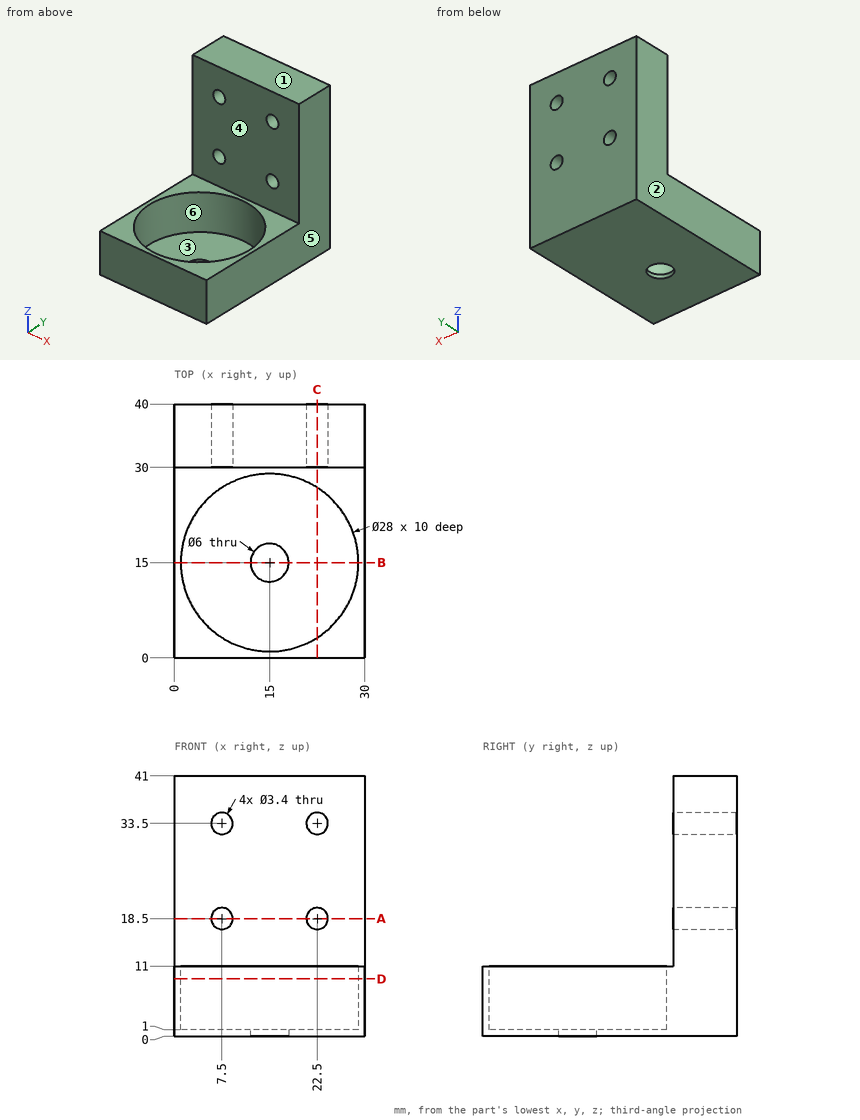
Drawing for the job (mm, zero at the part's lowest x, y, z). A direction names the side the tool comes from. Give positions to 0.01 mm unless a question says otherwise; leave off trailing zeros. Loops run counter-clockwise (first coordinate to the right, second up) from the corner with the lowest first, then second, coordinate; pieces in that order, holes last.
Item 1: Mould opens along X. For the marked faces 1, 2 and 3 say: +X half, -X half, draft (parallel to the pull), parting line (faces both ways), or undercut.
Check values:
face 1: draft
face 2: -X half
face 3: undercut
Item 2: Which spindle directions (+Z, -Z, +X, -X, +Y, -Y) get a long thin tool onto all of the face, cutting with end or side? Do the marked faces 4, 5 and 6. Say none if no direction does.
Check values:
face 4: +Z, +X, -X, -Y
face 5: +Z, -Z, +X, +Y, -Y
face 6: +Z
Item 3: Slice it at D-D (z = 9). Write the cut outline in (x, y), plus the area to 3 significant figures.
Check values:
outline: (0, 0) - (30, 0) - (30, 40) - (0, 40) - close; hole circle Ø28 at (15, 15)
area: 584 mm2
Item 4: Drill centre lines: line 1 along X through (y, z) = (32.75, 18.5); line 2 along Y through (x, z) = (15, 0.75); line 3 along Z through (x, y) = (22, 37). Where is each one in solid material? Low to high.
Check values:
line 1: x = 0 to 5.8, 9.2 to 20.8, 24.2 to 30
line 2: y = 0 to 12, 18 to 40
line 3: z = 0 to 16.88, 20.12 to 31.88, 35.12 to 41
Item 5: Slice it at C-C (x = 22.5). Write the cut outline in (y, z), plus the area to 3 significant figures.
Check values:
outline: (0, 0) - (40, 0) - (40, 16.8) - (30, 16.8) - (30, 11) - (26.82, 11) - (26.82, 1) - (3.18, 1) - (3.18, 11) - (0, 11) - close; (30, 20.2) - (40, 20.2) - (40, 31.8) - (30, 31.8) - close; (30, 35.2) - (40, 35.2) - (40, 41) - (30, 41) - close
area: 436 mm2
Item 6: Slice it at B-B (y = 15). Write the cut outline in (x, z).
Check values:
outline: (0, 0) - (12, 0) - (12, 1) - (1, 1) - (1, 11) - (0, 11) - close; (18, 0) - (30, 0) - (30, 11) - (29, 11) - (29, 1) - (18, 1) - close
Item 7: Drop flat-ended pins along their axis: P1, Ø5, axis at x = 3, y = 7, coming from the +Z side; P2, Ø9, axis at x = 22.5, y = 18.5, coming from the +Z side; P3, Ø4.5, axis at x = 22.5, z = 33.5, coming from the -Y side; P4, Ø3, axis at y = 33.5, z = 16, coming from the -X side. Give the stop position or say it passes through.
Check values:
P1: stops at z = 11
P2: stops at z = 1
P3: stops at y = 30
P4: stops at x = 0
Item 8: Slice it at A-A (z = 18.5). Write the cut outline in (x, y), plus the area to 3 significant figures.
Check values:
outline: (0, 30) - (5.8, 30) - (5.8, 40) - (0, 40) - close; (9.2, 30) - (20.8, 30) - (20.8, 40) - (9.2, 40) - close; (24.2, 30) - (30, 30) - (30, 40) - (24.2, 40) - close
area: 232 mm2
